```python
from build123d import *

# Parameters (mm, degrees)
F0_W     = 15
F0_H     = 20
F0_R     = 2
F1_DEPTH = 30
F2_W     = 0.55
F2_H     = 16.774644
F3_DEPTH = 15


with BuildPart() as f1:
    # F0 (on Front) → F1 (new body)
    with BuildSketch(Plane.XZ):
        with Locations((0, -1.499573)):
            Rectangle(F0_W, F0_H)
        Circle(F0_R, mode=Mode.SUBTRACT)
    extrude(amount=F1_DEPTH)

    # F2 (on face) → F3 (cut, through all)
    with BuildSketch(Plane.YZ.offset(7.5)):
        with Locations((-20.075855, 0.113105)):
            Rectangle(F2_W, F2_H)
    extrude(amount=-F3_DEPTH, mode=Mode.SUBTRACT)


solid = f1.part
```
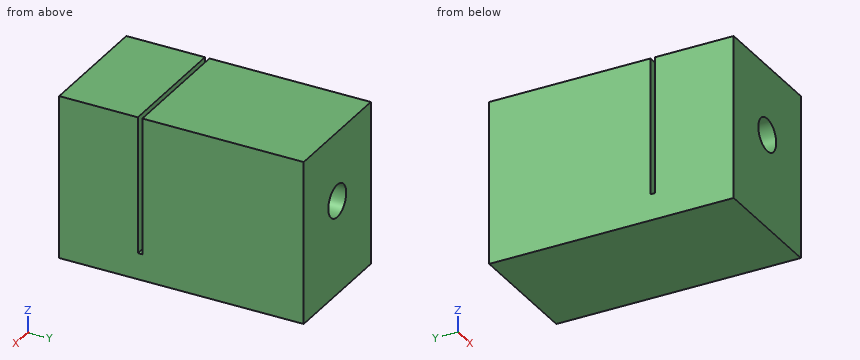
Here's how the part is built. I have some questions about the finished solid (model axes, mm). Give positions to 0.01 mm unless a question says otherwise; leave off trailing zeros. Write each loop counter-clockwise with the first axis right and the second up, starting at its lowest first coordinate (ties: lowest second). Pieces come first, ordered by that corner, then holes. Notation, with made-up numbers: M -11.75,-20.5 L 4.25,-20.5 A20 ccw 4.25,-16.5 Z; hole C 53,63 d2. An arc over 180 degrees is marked long. Put each result on its own line as item: value. Start each with the question number.
Item 1: I need wall thicknesses on L1, parallel to Y at x = 0, z = 5; L2, parallel to Z at x = 0, y = -5.75; L3, parallel to X at y = -13, z = 0. Which ranges of each line are inside material? Lowest first, please. Write a range as from..to.
Item 2: If we section it at B-B, the plane x = 0: Write out the boundary of the cut face in (y, z), then the cut area to 3 significant figures.
Item 3: If we section it at D-D, the plane x = -4: Write out the boundary of the cut face in (y, z), then the cut area to 3 significant figures.
Item 4: If we section it at C-C, the plane z = 5.75: Write out the boundary of the cut face in (x, y), then the cut area to 3 significant figures.
Item 5: If we section it at A-A, the plane z = 0: Write out the boundary of the cut face in (x, y), then the cut area to 3 significant figures.
Values:
1. L1: -30..-20.35, -19.8..0
1. L2: -11.5..-2, 2..8.5
1. L3: -7.5..-2, 2..7.5
2. outline: M -30,-11.5 L 0,-11.5 L 0,-2 L -19.8,-2 L -19.8,-8.27 L -20.35,-8.27 L -20.35,-2 L -30,-2 Z; M -30,2 L -20.35,2 L -20.35,8.5 L -30,8.5 Z; M -19.8,2 L 0,2 L 0,8.5 L -19.8,8.5 Z
2. area: 473 mm²
3. outline: M -30,-11.5 L 0,-11.5 L 0,8.5 L -19.8,8.5 L -19.8,-8.27 L -20.35,-8.27 L -20.35,8.5 L -30,8.5 Z
3. area: 591 mm²
4. outline: M -7.5,-30 L 7.5,-30 L 7.5,-20.35 L -7.5,-20.35 Z; M -7.5,-19.8 L 7.5,-19.8 L 7.5,0 L -7.5,0 Z
4. area: 442 mm²
5. outline: M -7.5,-30 L -2,-30 L -2,-20.35 L -7.5,-20.35 Z; M -7.5,-19.8 L -2,-19.8 L -2,0 L -7.5,0 Z; M 2,-30 L 7.5,-30 L 7.5,-20.35 L 2,-20.35 Z; M 2,-19.8 L 7.5,-19.8 L 7.5,0 L 2,0 Z
5. area: 324 mm²
